Geometry: see drawing. Coordinates: mm, zero at the bounding-box minimum. A direction names the side the tool comes from. Give positions to 0.01 mm unless a question says otherwise; leave off trailing zeros. Loops run counter-clockwise (first coordinate to the right, second up) from the corner with the lowest first, then second, coordinate; pieces in that order, holes last. Notation, with made-up numbers: (36.5, 26.25) -> (40.5, 26.25) arc R20 cw to (40.5, 30.25) -> close; hole circle Ø4 at (-35.5, 3). An arc over 180 degrees is marked (long way). Answer in a Markdown table with one row per item. Add a question column.
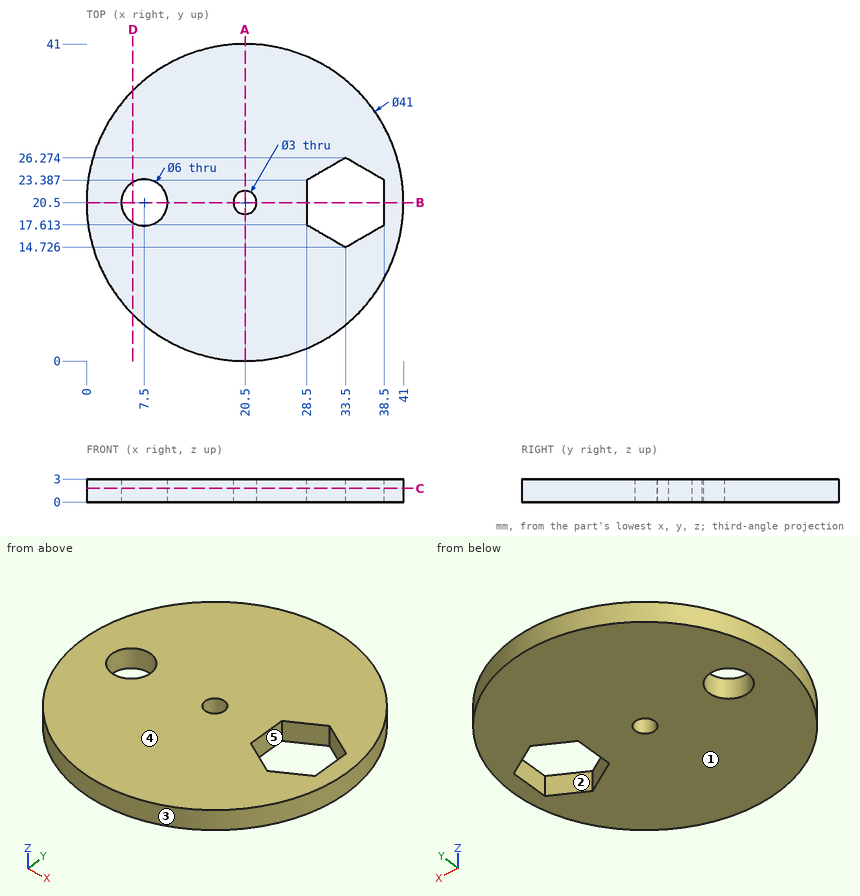
1) Reachability of the marked faces 1 and 2 from +Z, -Z, +X, -X, +Y, -Y: full face, straight path, thin tool, end or side. Return the list, or none.
2) Material intervals for line 1 along X through (y, z) = (20, 2.8) (1 decimal); line 2 along Y through (x, z) = (20.5, 1.45); line 3 along Y through (x, z) = (7.5, 2.45), sorted ascending.
3) Section B-B on y = 20.5. Output: boundary loops of the cut face in (x, z).
4) Section C-C on z = 1.8. Output: boundary loops of the cut face in (x, y).
5) Pin query (flat end, axial travel): pin 1 (1.5 mm diameter, centred on y = 19.5, z = 2, fed in from +X); pin 2 (1 mm diameter, centred on x = 23, z = 1, fed in from -Y); pin 3 (5 mm diameter, centred on x = 7.5, y = 20.5, fed in from -Z); pin 4 (1.5 mm diameter, centred on y = 19.5, z = 1, fed in from -X). Return the tip coordinate at first contact, or that it passes through.
6) Section D-D on x = 6. Output: boundary loops of the cut face in (y, z).
7) Pull-direction query (Y, two-part tool) for the marked faces 3, 4 and 5; classes: +Y half, -Y half, draft (parallel to the pull), parting line (faces both ways), or undercut.
8) Section A-A on x = 20.5. Output: boundary loops of the cut face in (y, z), and give its area (3 significant figures).
Working result:
| question | item | result |
|---|---|---|
| 1 | face 1 | -Z, +X, -X, +Y, -Y |
| 1 | face 2 | +Z, -Z |
| 2 | line 1 | x = 0 to 4.5, 10.5 to 19.1, 21.9 to 28.5, 38.5 to 41 |
| 2 | line 2 | y = 0 to 19, 22 to 41 |
| 2 | line 3 | y = 4.65 to 17.5, 23.5 to 36.35 |
| 3 | outline | (0, 0) -> (4.5, 0) -> (4.5, 3) -> (0, 3) -> close; (10.5, 0) -> (19, 0) -> (19, 3) -> (10.5, 3) -> close; (22, 0) -> (28.5, 0) -> (28.5, 3) -> (22, 3) -> close; (38.5, 0) -> (41, 0) -> (41, 3) -> (38.5, 3) -> close |
| 4 | outline | circle Ø41 at (20.5, 20.5); hole circle Ø6 at (7.5, 20.5); hole circle Ø3 at (20.5, 20.5); hole (28.5, 17.61) -> (33.5, 14.73) -> (38.5, 17.61) -> (38.5, 23.39) -> (33.5, 26.27) -> (28.5, 23.39) -> close |
| 5 | pin 1 | stops at x = 41 |
| 5 | pin 2 | stops at y = 0.1 |
| 5 | pin 3 | passes through |
| 5 | pin 4 | stops at x = 0 |
| 6 | outline | (6.01, 0) -> (17.9, 0) -> (17.9, 3) -> (6.01, 3) -> close; (23.1, 0) -> (34.99, 0) -> (34.99, 3) -> (23.1, 3) -> close |
| 7 | face 3 | parting line |
| 7 | face 4 | draft |
| 7 | face 5 | undercut |
| 8 | outline | (0, 0) -> (19, 0) -> (19, 3) -> (0, 3) -> close; (22, 0) -> (41, 0) -> (41, 3) -> (22, 3) -> close |
| 8 | area | 114 mm2 |
